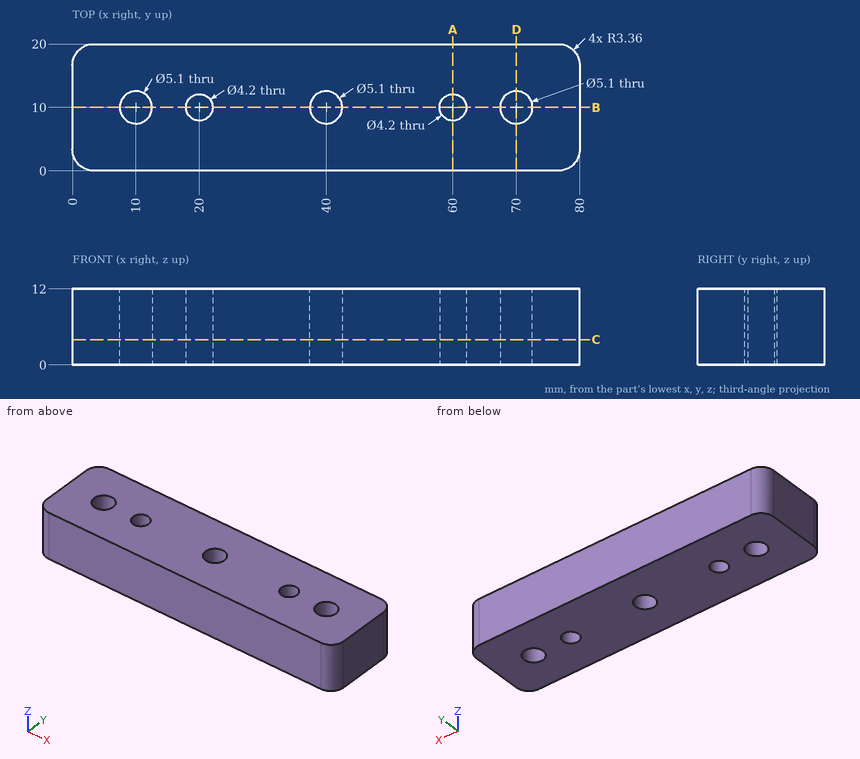
Here's the drawing with two shaded views (mm, measured from the low corner). I have some questions. Give positions to 0.01 mm unless a question says otherwise; leave off trailing zeros. Order: outer loops, then holes, each group sorted by start corner. A loop starts at its lowest first (then second) coordinate and runs counter-clockwise, first axis right, second up. Notation, with made-up numbers: M 24,-22.5 L 36,-22.5 A16 ccw 36,-14.5 Z; hole C -9.75,-25.75 d7. An arc over 180 degrees is marked long. Answer as a JSON object with one key per item and string values. Group by question number.
1) Please list where these lines run through material, in increasing order: L1, parallel to X at y = 7.75, z = 5.5; L2, parallel to Y at x = 40, z = 3.75; L3, parallel to X at y = 8.75, z = 4.5. Write a range as [from, to].
2) Suppose I cut it at A-A, the plane x = 60. Write out the boundary of the cut face in (y, z), plus the area to 3 significant figures.
3) Suppose I cut it at B-B, the plane y = 10. Write out the boundary of the cut face in (x, z).
4) Suppose I cut it at D-D, the plane x = 70. Write out the boundary of the cut face in (y, z).
5) Suppose I cut it at C-C, the plane z = 4. Write out the boundary of the cut face in (x, y), plus the area to 3 significant figures.
6) I'm going to push a flat-ended pin straight in: pin 1 Ø3.5 at (x, y) = (60, 10) entering from -Z. Where does the tip first touch, or does it pass through?
Results found:
{
 "1": {"L1": "[0, 8.8], [11.2, 38.8], [41.2, 68.8], [71.2, 80]", "L2": "[0, 7.45], [12.55, 20]", "L3": "[0, 7.78], [12.22, 18.31], [21.69, 37.78], [42.22, 58.31], [61.69, 67.78], [72.22, 80]"},
 "2": {"outline": "M 0,0 L 7.9,0 L 7.9,12 L 0,12 Z; M 12.1,0 L 20,0 L 20,12 L 12.1,12 Z", "area": "190 mm²"},
 "3": {"outline": "M 0,0 L 7.45,0 L 7.45,12 L 0,12 Z; M 12.55,0 L 17.9,0 L 17.9,12 L 12.55,12 Z; M 22.1,0 L 37.45,0 L 37.45,12 L 22.1,12 Z; M 42.55,0 L 57.9,0 L 57.9,12 L 42.55,12 Z; M 62.1,0 L 67.45,0 L 67.45,12 L 62.1,12 Z; M 72.55,0 L 80,0 L 80,12 L 72.55,12 Z"},
 "4": {"outline": "M 0,0 L 7.45,0 L 7.45,12 L 0,12 Z; M 12.55,0 L 20,0 L 20,12 L 12.55,12 Z"},
 "5": {"outline": "M 0,3.36 A3.36 ccw 3.36,0 L 76.64,0 A3.36 ccw 80,3.36 L 80,16.64 A3.36 ccw 76.64,20 L 3.36,20 A3.36 ccw 0,16.64 Z; hole C 10,10 d5.1; hole C 20,10 d4.2; hole C 40,10 d5.1; hole C 60,10 d4.2; hole C 70,10 d5.1", "area": "1,500 mm²"},
 "6": {"pin 1": "through"}
}
